```python
from build123d import *

# Parameters (mm, degrees)
SKETCH_1_W               = 64
SKETCH_1_H               = 32
EXTRUDE_1_DEPTH          = 8
EXTRUDE_START            = 8
SKETCH_2_R               = 3
EXTRUDE_2_DEPTH          = 8
EXTRUDE_3_REACH          = 72.029
SKETCH_3_R               = 3
CUT_EXTRUDE_1_REACH      = 72.029
CUT_EXTRUDE_1_END_RADIUS = 3
SKETCH_4_R               = 1.5
CUT_EXTRUDE_START        = -8
SKETCH_5_R               = 5
CUT_EXTRUDE_3_DEPTH      = 69.728905803


with BuildPart() as part:
    # 草图1 → 凸台-拉伸1 (new body)
    with BuildSketch(Plane(origin=(0, 0, 0), x_dir=(1, 0, 0), z_dir=(0, 1, 0))):
        Rectangle(SKETCH_1_W, SKETCH_1_H)
    extrude(amount=EXTRUDE_1_DEPTH)

    # 草图2 → 凸台-拉伸2 (add)
    with BuildSketch(Plane(origin=(0, 0, 0), x_dir=(0, 0, -1), z_dir=(1, 0, 0)).offset(EXTRUDE_START)):
        with BuildLine():
            Line((-16, 8), (-16, 14))
            Line((-16, 14), (13.44586918, 39.552706084))
            ThreePointArc((13.44586918, 39.552706084), (26.611734227, 39.502331005), (28.316651221, 26.447224796))
            Line((28.316651221, 26.447224796), (16, 8))
            Line((16, 8), (-16, 8))
        make_face()
        with Locations((20, 32)):
            Circle(SKETCH_2_R, mode=Mode.SUBTRACT)
    extrude_2 = extrude(amount=EXTRUDE_2_DEPTH)

    # 凸台-拉伸3: up to this plane
    extrude_3_end = Plane(origin=(16, 14, 16), z_dir=(0, -0.7552706084274633, -0.6554130819915097))
    # 草图3 → 凸台-拉伸3 (add, up to the surface)
    with BuildSketch(Plane.XY.offset(16), mode=Mode.PRIVATE) as extrude_3_sk1:
        with Locations((12, 31.770444903)):
            Circle(SKETCH_3_R)
    extrude_3_tool1 = split(extrude(extrude_3_sk1.sketch, amount=-EXTRUDE_3_REACH, mode=Mode.PRIVATE), bisect_by=extrude_3_end, keep=Keep.BOTH, mode=Mode.PRIVATE)
    extrude_3 = extrude_3_tool1.solids().sort_by_distance((12, 31.770445, 16))[0]
    add(extrude_3)

    # 切除-拉伸1: up to this cylinder (the profile starts outside it)
    cut_extrude_1_end = Plane(origin=(12, 32, -20), z_dir=(-1, 0, 0)) * Cylinder(CUT_EXTRUDE_1_END_RADIUS, 151.058, mode=Mode.PRIVATE)
    # 草图4 → 切除-拉伸1 (cut, up to the surface)
    with BuildSketch(Plane.XY.offset(16), mode=Mode.PRIVATE) as cut_extrude_1_sk1:
        with Locations((12, 31.770444903)):
            Circle(SKETCH_4_R)
    cut_extrude_1_tool1 = extrude(cut_extrude_1_sk1.sketch, amount=-CUT_EXTRUDE_1_REACH, mode=Mode.PRIVATE) - cut_extrude_1_end
    cut_extrude_1 = cut_extrude_1_tool1.solids().sort_by_distance((12, 31.770445, 16))[0]
    add(cut_extrude_1, mode=Mode.SUBTRACT)

    # 镜向1: 凸台-拉伸2, 凸台-拉伸3, 切除-拉伸1 across plane
    add(extrude_2.mirror(Plane(origin=(0, 0, 0), x_dir=(0, 0, 1), z_dir=(1, 0, 0))))
    add(extrude_3.mirror(Plane(origin=(0, 0, 0), x_dir=(0, 0, 1), z_dir=(1, 0, 0))))
    add(cut_extrude_1.mirror(Plane(origin=(0, 0, 0), x_dir=(0, 0, 1), z_dir=(1, 0, 0))), mode=Mode.SUBTRACT)

    # 草图5 → 切除-拉伸3 (cut)
    with BuildSketch(Plane(origin=(0, 0, 0), x_dir=(1, 0, 0), z_dir=(0, 1, 0)).offset(CUT_EXTRUDE_START)):
        with Locations(Location((-25, 0, 0), (0, 0, 270))):
            Circle(SKETCH_5_R)
    cut_extrude_3 = extrude(amount=CUT_EXTRUDE_3_DEPTH, mode=Mode.SUBTRACT)

    # 镜向2: 切除-拉伸3 across plane
    add(cut_extrude_3.mirror(Plane(origin=(0, 0, 0), x_dir=(0, 0, 1), z_dir=(1, 0, 0))), mode=Mode.SUBTRACT)


solid = part.part
```
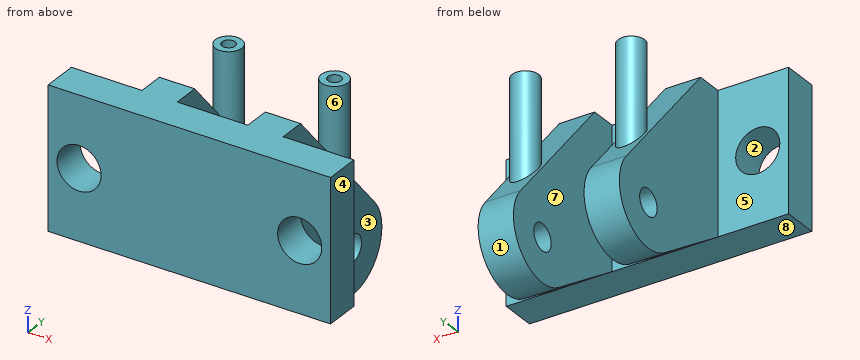
Geometry: final body of the model. Coordinates: model frame, mm. Face numbers are marked on the shaded views. A direction names the side the tool comes from. Round coordinates to 2 decimals unless told otherwise and drop trailing zeros. Order: outer loops, then holes, each group sorted by start corner. A loop starts at its lowest first (then second) coordinate and runs counter-clockwise, first axis right, second up. Notation, with made-up numbers: (1.25, 30.5) -> (39.25, 30.5) arc R7 cw to (39.25, 43.5) -> close; hole circle Ø3 at (28.25, 52). An arc over 180 degrees is marked (long way). Use CSV: the item, a comma, the result in double quotes. Start each with the question number.
1) First-contact query: pin 1 Ø10 at (x, z) = (4.5, 3) entering from +Y; pin 2 Ø17 at (y, z) = (26.5, -16.5) entering from -X; pin 3 Ø6 at (x, y) = (11, 24.5) entering from +Z; pin 4 Ø9 at (x, z) = (25, 0) entering from +Y. Flat tips, straight axial feed; report the tip coordinate or a pass-through.
2) Draft query along X for the marked faces 1, 2 and 3. Return one class per face: +X half, -X half, draft (parallel to the pull), parting line (faces both ways), or undercut.
3) Section C-C (z = 9). Return the cut outline in (x, y).
4) Section A-A (z = 0). Return the cut outline in (x, y).
5) Section D-D (z = -20). Return the cut outline in (x, y), and give its area (3 significant figures).
6) Set-up query: the marked faces 4, 5, 6, 7 and 8. Return all of +Z, -Z, +X, -X, +Y, -Y with unobstructed straight access to the full face (end or side cutting, diameter ignored); none if empty.
7) Material intervals for line 1 along X through (y, z) = (4.5, 0); line 2 along Z through (x, y) = (-25, 6.25); line 3 along X through (y, z) = (18, -3), sorted ascending. Write a range as from..to.
8) Section B-B (y = 22). Return the cut outline in (x, z).
Returned:
1,pin 1,"stops at y = 33.43"
1,pin 2,"stops at x = -16"
1,pin 3,"stops at z = 7.36"
1,pin 4,"passes through"
2,face 1,"draft"
2,face 2,"undercut"
2,face 3,"+X half"
3,outline,"(-32, 0) -> (32, 0) -> (32, 8) -> (16, 8) -> (16, 20.07) -> (8, 20.07) -> (8, 8) -> (-8, 8) -> (-8, 20.07) -> (-16, 20.07) -> (-16, 8) -> (-32, 8) -> close; circle Ø6 at (-12, 31.77); circle Ø6 at (12, 31.77); hole circle Ø3 at (-12, 31.77); hole circle Ø3 at (12, 31.77)"
4,outline,"(-32, 0) -> (-30, 0) -> (-30, 8) -> (-32, 8) -> close; (-20, 0) -> (20, 0) -> (20, 8) -> (16, 8) -> (16, 27.88) -> (8, 27.88) -> (8, 8) -> (-8, 8) -> (-8, 27.88) -> (-16, 27.88) -> (-16, 8) -> (-20, 8) -> close; circle Ø6 at (-12, 31.77); circle Ø6 at (12, 31.77); (30, 0) -> (32, 0) -> (32, 8) -> (30, 8) -> close; hole circle Ø3 at (-12, 31.77); hole circle Ø3 at (12, 31.77)"
5,outline,"(-16, 13.99) -> (-8, 13.99) -> (-8, 29) -> (-16, 29) -> close; (-16, 35) -> (-8, 35) -> (-8, 42) -> (-16, 42) -> close; (8, 13.99) -> (16, 13.99) -> (16, 29) -> (8, 29) -> close; (8, 35) -> (16, 35) -> (16, 42) -> (8, 42) -> close"
5,area,"352 mm²"
6,face 4,"+Z, -Z, +X, +Y, -Y"
6,face 5,"+Z, -Z, -X, +Y"
6,face 6,"+Z"
6,face 7,"+Z, -Z, +Y"
6,face 8,"-Z, +X, -X, -Y"
7,line 1,"x = -32..-30, -20..20, 30..32"
7,line 2,"z = -16..-5, 5..16"
7,line 3,"x = -16..-8, 8..16"
8,outline,"(-16, -25.35) -> (-8, -25.35) -> (-8, 6.78) -> (-16, 6.78) -> close; (8, -25.35) -> (16, -25.35) -> (16, 6.78) -> (8, 6.78) -> close"
